Here's the drawing with two shaded views (mm, measured from the low corner). I have some questions. A direction names the side the tool comes from. Give positions to 0.01 mm unless a question says otherwise; leave off trailing zeros. Write each loop counter-clockwise with the first axis right and the second up, starting at its lowest first coordinate (ties: lowest second). Pieces come first, ordered by that corner, then holes. Notation, with made-up numbers: M 49.5,16 L 96.5,16 A24 cw 96.5,37 Z; hole C 15,17.5 d11. An arc over 180 degrees is marked long. Answer as CSV lines item,"result". Start each with the question number.
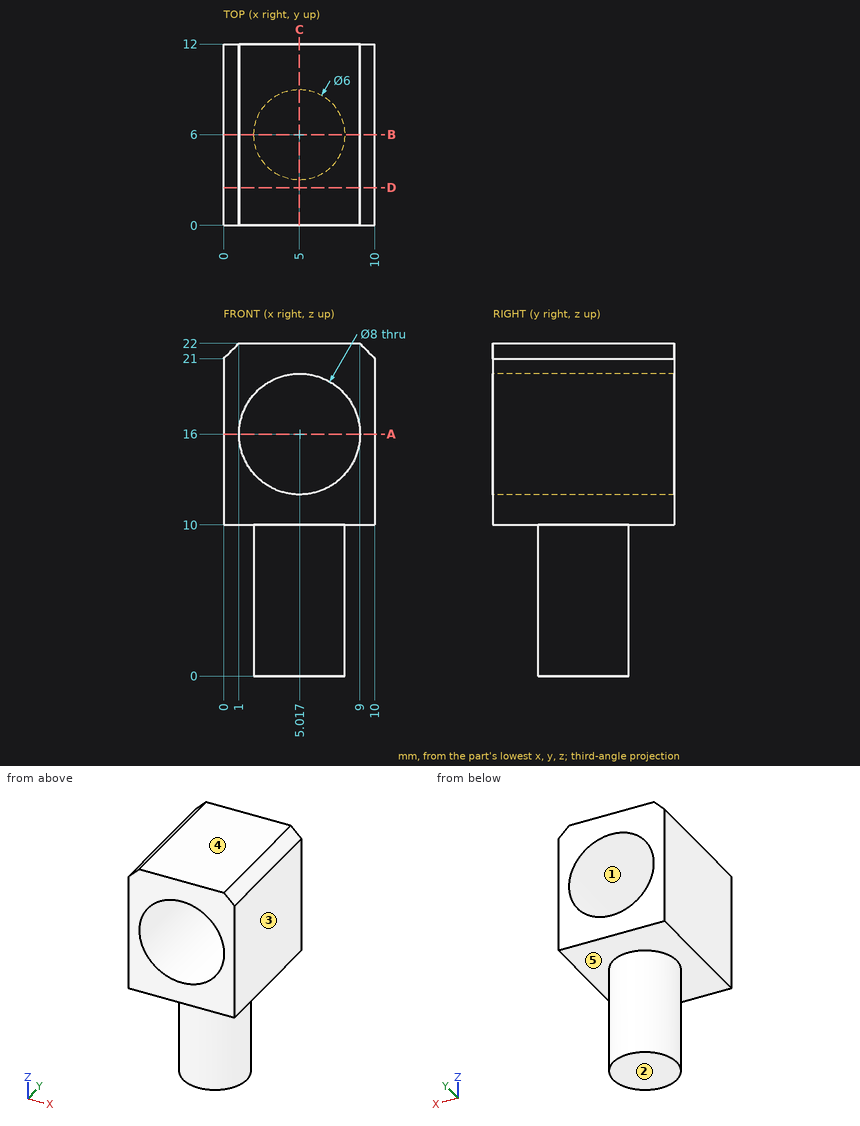
1. Imagine slicing it at D-D, the plane y = 2.5. Please give me the cut outline in (x, z).
2. Imagine slicing it at C-C, the plane x = 5. Please give me the cut outline in (y, z), plus the area to 3 significant figures.
3. Imagine slicing it at B-B, the plane y = 6. Please give me the cut outline in (x, z).
4. Thinking about a two-plate mould opening in Z: for the marked faces 1, 2 and 3, which applies, pulls with the +Z half, pulls with the -Z half, needs draft (parallel to the pull), parting line crosses it, or undercut?
5. Please list where these lines run through material, in increasing order: line 1 (X direction, y = 3, z = 16); line 2 (X direction, y = 2, z = 13.5) (1 decimal); line 3 (Z direction, x = 2.5, y = 9.5).
6. Imagine slicing it at A-A, the plane z = 16. Please give me the cut outline in (x, y), plus the area to 3 significant figures.
7. On a 3-axis mill with a long thin cutter (end or side, diameter ignored), from which of +Z, -Z, +X, -X, +Y, -Y can I reach the whole of each face in a straight line? I mean the marked faces 4 and 5. Say none if no direction works.
8. Will this pin go through, and if not, where does the flat tip stop? P1, Ø3, axis at y = 3.5, z = 5, coming from the -X side.
Solutions:
1,outline,"M 0,10 L 10,10 L 10,21 L 9,22 L 1,22 L 0,21 Z; hole C 5.02,16 d8"
2,outline,"M 0,10 L 3,10 L 3,0 L 9,0 L 9,10 L 12,10 L 12,12 L 0,12 Z; M 0,20 L 12,20 L 12,22 L 0,22 Z"
2,area,"108 mm²"
3,outline,"M 0,10 L 2,10 L 2,0 L 8,0 L 8,10 L 10,10 L 10,21 L 9,22 L 1,22 L 0,21 Z; hole C 5.02,16 d8"
4,face 1,"undercut"
4,face 2,"pulls with the -Z half"
4,face 3,"needs draft"
5,line 1,"0 to 1.02, 9.02 to 10"
5,line 2,"0 to 1.9, 8.1 to 10"
5,line 3,"10 to 12.89, 19.11 to 22"
6,outline,"M 0,0 L 1.02,0 L 1.02,12 L 0,12 Z; M 9.02,0 L 10,0 L 10,12 L 9.02,12 Z"
6,area,"24.0 mm²"
7,face 4,"+Z, +X, -X, +Y, -Y"
7,face 5,"-Z"
8,P1,"x = 2.17"
